from build123d import *

# Parameters (mm, degrees)
SKETCH1_W           = 20
SKETCH1_H           = 12
SKETCH1_R           = 1.6
BOSS_EXTRUDE1_DEPTH = 44
SKETCH2_W           = 36
SKETCH2_H           = 15
CUT_EXTRUDE1_DEPTH  = 51.049975025
CHAMFER1_SIZE       = 2
FILLET1_R           = 1
SKETCH3_R           = 2.15
CUT_EXTRUDE2_DEPTH  = 48.549973712


with BuildPart() as part:
    # Sketch1 → Boss-Extrude1 (new body)
    # profile 1 of 2: a face of its own
    with BuildSketch(Plane(origin=(0, 0, 0), x_dir=(0, 0, -1), z_dir=(1, 0, 0))):
        Rectangle(SKETCH1_W, SKETCH1_H)
    # profile 2 of 2: a face of its own
    with BuildSketch(Plane(origin=(0, 0, 0), x_dir=(0, 0, -1), z_dir=(1, 0, 0))):
        with BuildLine():
            ThreePointArc((-2.529576231, 12.098587435), (0, 13), (2.529576231, 12.098587435))
            Line((2.529576231, 12.098587435), (10, 6))
            Line((10, 6), (-10, 6))
            Line((-10, 6), (-2.529576231, 12.098587435))
        make_face()
        with Locations((0, 9)):
            Circle(SKETCH1_R, mode=Mode.SUBTRACT)
    extrude(amount=BOSS_EXTRUDE1_DEPTH)

    # Sketch2 → Cut-Extrude1 (cut, through all)
    with BuildSketch(Plane.XY.offset(10)):
        with Locations((22, 5.5)):
            Rectangle(SKETCH2_W, SKETCH2_H)
    extrude(amount=-CUT_EXTRUDE1_DEPTH, mode=Mode.SUBTRACT)

    # Chamfer1
    chamfer1_edges = [part.edges().sort_by_distance(p)[0] for p in [
        (4, -2, 0),
        (40, -2, 0),
    ]]
    chamfer(chamfer1_edges, length=CHAMFER1_SIZE)

    # Fillet1
    fillet1_edges = [part.edges().sort_by_distance(p)[0] for p in [
        (0, 9.049293718, -6.264788115),
        (0, 0, -10),
        (44, 9.049293718, -6.264788115),
        (42, 6, 10),
        (44, 13, 0),
        (44, 9.049293718, 6.264788115),
        (2, 6, 10),
        (44, 0, 10),
        (4, 9.049293718, -6.264788115),
        (4, 3, -10),
        (4, 13, 0),
        (4, 9.049293718, 6.264788115),
        (40, 9.049293718, -6.264788115),
        (40, 9.049293718, 6.264788115),
        (40, 13, 0),
        (4, 3, 10),
        (40, 3, -10),
        (40, 3, 10),
        (22, -2, 10),
        (22, -2, -10),
        (6, -2, 0),
        (38, -2, 0),
        (39, -1, 10),
        (39, -1, -10),
        (5, -1, 10),
        (5, -1, -10),
        (0, 0, 10),
        (44, 0, -10),
        (0, 9.049293718, 6.264788115),
        (0, 13, 0),
    ]]
    fillet(fillet1_edges, radius=FILLET1_R)

    # Sketch3 → Cut-Extrude2 (cut, through all)
    with BuildSketch(Plane(origin=(0, -2, 0), x_dir=(1, 0, 0), z_dir=(0, 1, 0))):
        with Locations(Location((12, 0, 0), (0, 0, 270))):
            Circle(SKETCH3_R)
        with Locations(Location((32, 0, 0), (0, 0, 270))):
            Circle(SKETCH3_R)
    extrude(amount=-CUT_EXTRUDE2_DEPTH, mode=Mode.SUBTRACT)


solid = part.part
Model file for the job. Use its own axes, mm. A direction names the side the tool comes from. Give positions to 0.01 mm unless a question says otherwise; leave off trailing zeros. Order: outer loops, then holes, each group sorted by start corner. A loop starts at its lowest first (then second) coordinate and runs counter-clockwise, first axis right, second up. Notation, with made-up numbers: (5.25, 43) - (62.25, 43) arc R34 ccw to (62.25, 82) - close; hole circle Ø10 at (62, 23). An arc over 180 degrees is marked (long way). Return JSON: item names as keys, results as strings.
1) Pull direction Z, two halves, no side cores. Call faces 1 (the cylindrical face through (33.81, -3.97, 1.16)), 2 (the cylindrical face through (2, 13, 0)), 3 (the cylindrical face through (41.97, 7.44, 0.35)), 4 (the flat face through (44, 1, 0)): pulls with the +Z half, pulls with the -Z half, needs draft (parallel to the pull), parting line crosses it, or undercut.
Geometry says:
{"face 1": "undercut", "face 2": "parting line crosses it", "face 3": "undercut", "face 4": "needs draft"}
2) Probe line 1 (X direction, y = -4.85, z = 0); line 2 (X direction, y = 5.5, z = -2); line 3 (Y direction, x = 30.5, z = 7.5). List the from-to ranges inside material, lowest first. Write a range as from..to.
Geometry says:
{"line 1": "0..9.85, 14.15..29.85, 34.15..44", "line 2": "0..4, 40..44", "line 3": "-6..-2"}
3) Cut at A-A, the plane x = 32. Give the cut face in (y, z).
Geometry says:
{"outline": "(-6, -10) - (-3, -10) arc R1 ccw to (-2, -9) - (-2, -2.15) - (-6, -2.15) - close; (-6, 2.15) - (-2, 2.15) - (-2, 9) arc R1 ccw to (-3, 10) - (-6, 10) - close"}
4) 3-axis set-ups, long thin cutter, end or side, ignore diameter. For faces 5 (the cylindrical face through (0.301, 0.084, -9.715)), 6 (the flat face through (39, -1, 0)), 7 (the cylindrical face through (3.699, 2.838, -9.715)), 8 (the cylindrical face through (40.285, 9.007, 5.841)): which of +Z, -Z, +X, -X, +Y, -Y reach the whole face in a straight line?
Geometry says:
{"face 5": "-Z, -X, +Y, -Y", "face 6": "+Z, -Z, +Y", "face 7": "-Z, +Y", "face 8": "+Z, +Y"}
5) Cut at B-B, the plane x = 15. Give the cut face in (y, z).
Geometry says:
{"outline": "(-6, -10) - (-3, -10) arc R1 ccw to (-2, -9) - (-2, 9) arc R1 ccw to (-3, 10) - (-6, 10) - close"}
6) Flat gauge pins, fed straight in: P1, Ø3.5, axis at y = 9, z = 0, coming from the -X side; P2, Ø4, axis at x = 20, z = -7, coming from the +Y side. Where does each tip first touch, or does it go through?
Geometry says:
{"P1": "x = 0", "P2": "y = -2"}
7) Cut at C-C, the plane y = 9. Count the separate pieces of the cut face and the enclosed holes in it, plus the area to 3 significant figures.
Geometry says:
{"separate pieces": "4", "enclosed holes": "0", "area": "72.9 mm²"}
